The listing builds one solid part. Answer for the finished solid, in the listing's coordinates (mm). A direction names the side the tool comes from. Coordinates: 2 decimals unless noted, no trailing zeros. Write each loop counter-clockwise with the first axis right and the second up, starting at its lowest first coordinate (ties: lowest second). Pieces come first, ordered by that corner, then holes.
from build123d import *

# Parameters (mm, degrees)
SKETCH1_R           = 35
BOSS_EXTRUDE1_DEPTH = 22
SKETCH2_R           = 18
BOSS_EXTRUDE2_DEPTH = 17
SKETCH3_R           = 10
BOSS_EXTRUDE3_DEPTH = 24
CUT_EXTRUDE1_START  = -2
SKETCH4_R           = 19
SKETCH4_R_2         = 18
CUT_EXTRUDE1_DEPTH  = 2


with BuildPart() as part:
    # Sketch1 → Boss-Extrude1 (new body)
    with BuildSketch(Plane(origin=(0, 0, 0), x_dir=(0, 0, -1), z_dir=(1, 0, 0))):
        Circle(SKETCH1_R)
    extrude(amount=BOSS_EXTRUDE1_DEPTH)

    # Sketch2 → Boss-Extrude2 (add)
    with BuildSketch(Plane(origin=(22, 0, 0), x_dir=(0, 0, -1), z_dir=(1, 0, 0))):
        Circle(SKETCH2_R)
    extrude(amount=BOSS_EXTRUDE2_DEPTH)

    # Sketch3 → Boss-Extrude3 (add)
    with BuildSketch(Plane(origin=(39, 0, 0), x_dir=(0, 0, -1), z_dir=(1, 0, 0))):
        Circle(SKETCH3_R)
    extrude(amount=BOSS_EXTRUDE3_DEPTH)

    # Sketch4 → Cut-Extrude1 (cut)
    with BuildSketch(Plane(origin=(22, 0, 0), x_dir=(0, 0, -1), z_dir=(1, 0, 0)).offset(CUT_EXTRUDE1_START)):
        Circle(SKETCH4_R)
        Circle(SKETCH4_R_2, mode=Mode.SUBTRACT)
    extrude(amount=CUT_EXTRUDE1_DEPTH, mode=Mode.SUBTRACT)


solid = part.part
Q1. The part is cut by section D-D, the plane z = 12. Write down the section's boundary in (x, y).
Answers below:
outline: (0, -32.88) - (22, -32.88) - (22, -14.73) - (20, -14.73) - (20, -13.42) - (39, -13.42) - (39, 13.42) - (20, 13.42) - (20, 14.73) - (22, 14.73) - (22, 32.88) - (0, 32.88) - close
Q2. Given pin 1 (6 mm diameter, centred on x = 47, z = 6, fed in from +Y); pin 2 (2 mm diameter, centred on x = 35.5, y = -12, fed in from +Z); pin 3 (6 mm diameter, centred on x = 19, y = 9, fed in from +Z), each flat-ended and moving along its own axis, determine where each tip first touches the part or whether it passes through.
Answers below:
pin 1: stops at y = 9.54
pin 2: stops at z = 14.25
pin 3: stops at z = 34.48
Q3. The part is cut by section A-A, the plane z = 0. Write down the section's boundary in (x, y).
Answers below:
outline: (0, -35) - (22, -35) - (22, -19) - (20, -19) - (20, -18) - (39, -18) - (39, -10) - (63, -10) - (63, 10) - (39, 10) - (39, 18) - (20, 18) - (20, 19) - (22, 19) - (22, 35) - (0, 35) - close
Q4. Which of the six approach directions +Z, -Z, +X, -X, +Y, -Y give full straight-line access (tool end or side, diameter ignored) to faces 4 (the face through (22, -15, -15)), 5 (the face through (63, 0, 0))?
Answers below:
face 4: +X
face 5: +Z, -Z, +X, +Y, -Y
Q5. Determine the mould class of faces 1 (the face through (50.83, -9.76, 2.17)), 2 (the face through (20.986, -16.856, -8.767)), 3 (the face through (0, 0, 0)) for opening direction Y: released by +Y, released by -Y, zero draft, split by the parting line, or undercut.
Answers below:
face 1: split by the parting line
face 2: undercut
face 3: zero draft
Q6. The part is cut by section C-C, the plane x = 13. Write down the section's boundary in (y, z).
Answers below:
outline: circle Ø70 at (0, 0)
Q7. Find the intervals of material crossed by probe 1 along Y at (x, z) = (21, 0); probe 2 along X at (y, z) = (-5.5, -29.5); probe 3 along Y at (x, z) = (8, -1), in increasing order.
Answers below:
probe 1: y = -35 to -19, -18 to 18, 19 to 35
probe 2: x = 0 to 22
probe 3: y = -34.99 to 34.99
